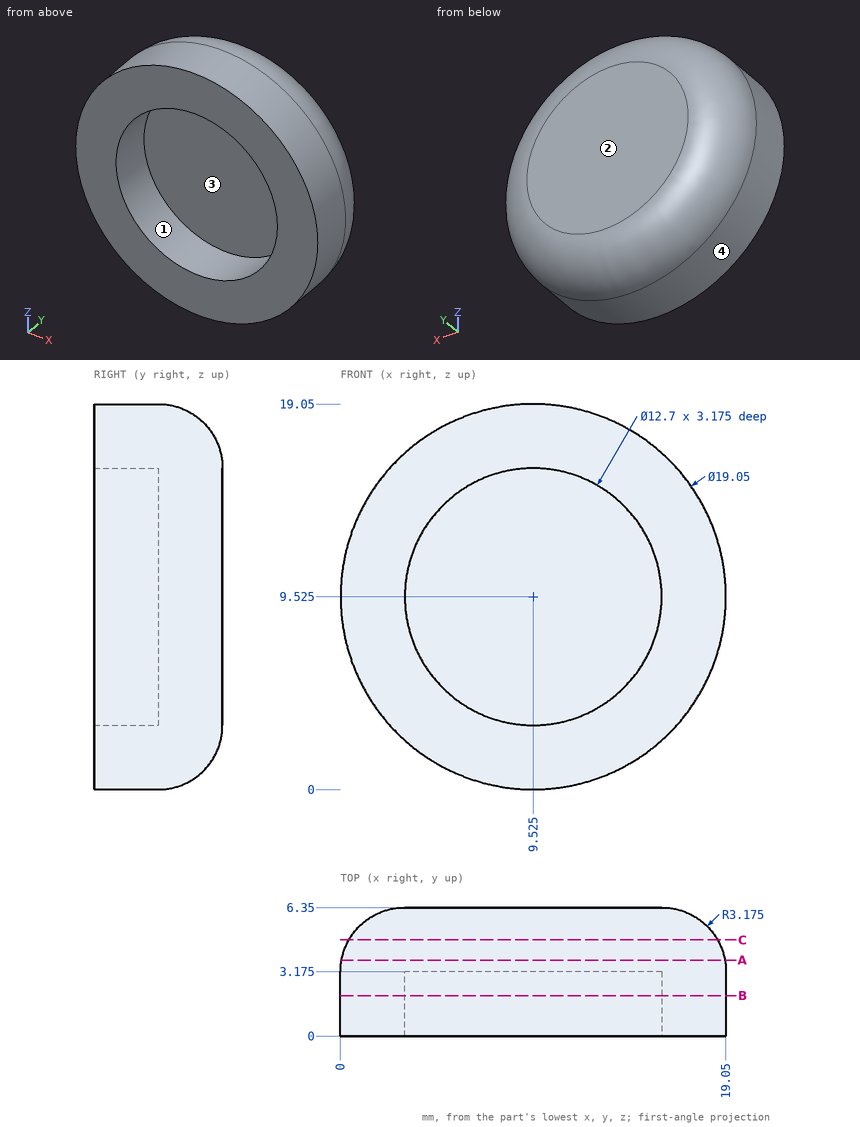
Geometry check sheet. Reference: drawing and pictorial views, mm from the part's lowest x, y, z. Give positions to 0.01 mm unless a question says otherwise; leave off trailing zeros. Write each loop counter-clockwise with the first axis right and the second up, starting at its lowest first coordinate (ties: lowest second). Pieces come first, ordered by that corner, then holes. Notation, with made-up numbers: M 0,31 L 53,31 A16 cw 53,51 Z; hole C -22.75,2 d10. An arc over 180 degrees is marked long. Answer as CSV lines item,"result". Start each with the question number.
Q1. Section check A-A, the plane y = 3.75. Record the cut outline in (x, z) (1 decimal), then the cut area to 3 significant figures.
Q2. Go/stop test with flat-tipped pins: pin 1 (2 mm diameter, centred on y = 1.5, z = 12.5, fed in from +X); pin 2 (1.5 mm diameter, centred on x = 13, y = 5.5, fed in from +Z); pin 3 (1 mm diameter, centred on y = 3, z = 10.5, fed in from -X). Record where each tip stops, or that it passes through.
Q3. Material ranges on L1, parallel to Y at x = 9.5, z = 10.75 (3 decimals); L2, parallel to Z at x = 10.75, y = 0.5; L3, parallel to Z at x = 4, y = 1.25 (3 decimals), recorded low to high.
Q4. Release check for a two-part mould opening along X. For the marked faces 1, 2, 3 and 4 record: pulls with the +X half, pulls with the -X half, needs draft (parallel to the pull), parting line crosses it, or undercut.
Q5. Section check B-B, the plane y = 2. Record the cut outline in (x, z) (3 decimals), then the cut area to 3 significant figures.
Q6. Section check C-C, the plane y = 4.75. Record the cut outline in (x, z) (3 decimals).
Geometry says:
1,outline,"C 9.5,9.5 d18.9"
1,area,"282 mm^2"
2,pin 1,"x = 18.84"
2,pin 2,"z = 18.02"
2,pin 3,"x = 0.01"
3,L1,"3.175 to 6.35"
3,L2,"0.08 to 3.29, 15.76 to 18.97"
3,L3,"1.766 to 6.395, 12.655 to 17.284"
4,face 1,"undercut"
4,face 2,"needs draft"
4,face 3,"undercut"
4,face 4,"parting line crosses it"
5,outline,"C 9.525,9.525 d19.05; hole C 9.525,9.525 d12.7"
5,area,"158 mm^2"
6,outline,"C 9.525,9.525 d18.214"
